Autodesk Inventor part; units mm, degrees
ref_plane "YZ Plane" through (0, 0, 0) normal (1, 0, 0) x (0, 1, 0)
ref_plane "XZ Plane" through (0, 0, 0) normal (0, 1, 0) x (-1, 0, 0)
ref_plane "XY Plane" through (0, 0, 0) normal (0, 0, 1) x (1, 0, 0)
sketch "Sketch1" plane through (0, 0, 0) normal (0, 1, 0) x (-1, 0, 0)
  line L0 (0, 0) -> (-2, 0)
  line L1 (-2, 0) -> (-3.1369, 0)
  line L2 (-3.1369, 0) -> (-3.1369, -16)
  line L3 (-3.1369, -16) -> (-1.7653, -16)
  line L4 (-1.7653, -16) -> (-1.7653, -18.3622)
  line L5 (-1.7653, -18.3622) -> (-3.1369, -18.3622)
  line L6 (-3.1369, -18.3622) -> (-3.1369, -19.3622)
  line L7 (-2, 0) -> (0, 0)
  line L8 (-2, 0) -> (0, 0)
  line L9 (-3.1369, -19.3622) -> (-3, -19.3622)
  line L10 (-3, -19.3622) -> (-3, -35.3622)
  line L11 (-3, -35.3622) -> (0, -35.3622)
  line L12 (0, -35.3622) -> (0, 0)
  dimension "d1" = 0
  dimension "d2" = 16
  dimension "d3" = 2.3622
  dimension "d6" = 3.1369
  dimension "d8" = 3
  dimension "d13" = 1
  dimension "d29" = 1.7653
  dimension "d30" = 16
revolve "Revolution1" add sketch "Sketch1" angle 360 about axis through (0, 0, -35.3622) along (0, 0, 1)
thread "Thread1"
sketch "Sketch3" plane through (0, 0, 0) normal (0, 0, 1) x (1, 0, 0)
  circle A0 centre (0, 0) radius 3.1369
  line L0 (-2.4166, -2) -> (2.4166, -2)
  line L1 (-2.5237, 1.8631) -> (2.5237, 1.8631)
  arc A1 (2.4166, -2) -> (2.5237, 1.8631) centre (0, 0) ccw
  arc A2 (-2.5237, 1.8631) -> (-2.4166, -2) centre (0, 0) ccw
  point P0 (0, 0)
  dimension "d36" = 5
extrude "Extrusion1" cut sketch "Sketch3" against normal blind 10 contours L1 A0
sketch "Sketch4" plane through (-2.5237, 1.8631, 0) normal (0, 1, 0) x (1, 0, 0)
  circle A0 centre (2.5237, 3) radius 1
  point P0 (2.5237, 0)
  dimension "d23" = 2
  dimension "d24" = 3
extrude "Extrusion2" cut sketch "Sketch4" against normal blind 10
thread "Thread2"
sketch "Sketch5" plane through (0, 0, -35.3622) normal (0, 0, -1) x (-1, 0, 0)
  circle A0 centre (0, 0) radius 3.1369
  line L0 (-2.5237, 1.8631) -> (2.5258, 1.8631)
  line L1 (2.5258, 1.8631) -> (2.5258, 4.5959)
  line L2 (2.5258, 4.5959) -> (-2.5237, 4.5959)
  line L3 (-2.5237, 4.5959) -> (-2.5237, 1.8631)
  point P0 (0, 0)
  dimension "d33" = 5
extrude "Extrusion3" cut sketch "Sketch5" against normal blind 16 contours L0 A0 | A0 L3 L2 L1 picked at (-0.6375, 2.3533)
properties part number "rod"
Geometry check sheet. Reference: the model listing, model coordinates, mm. A direction names the side the tool comes from. Give positions to 0.01 mm unless a question says otherwise; leave off trailing zeros. Order: outer loops, then holes, each group sorted by start corner. A loop starts at its lowest first (then second) coordinate and runs counter-clockwise, first axis right, second up. Notation, with made-up numbers: (-27, -11.5) - (2, -11.5) arc R7 cw to (2, -4.5) - close; hole circle Ø5 at (4, 49.5). An arc over 180 degrees is marked (long way). Write item = value, one per line. Start each with the question number.
1) Gauge pin test, flat ends, axial feed: pin 1 Ø3 at (x, y) = (-1, -0.5) entering from +Z; pin 2 Ø2.5 at (x, z) = (1, -28) entering from +Y; pin 3 Ø1 at (x, y) = (-1, 2.5) entering from +Z; pin 4 Ø1 at (x, z) = (-0.5, -24) entering from -Y. Record the tip position at first contact, or that the pin passes through.
2) Scan lines: L1, parallel to Z at x = -2.25, y = 0.5; L2, parallel to Z at x = -1.75, y = 2.5; L3, parallel to X at y = -0.6, z = -3. Record each from-to range of solid material in increasing order.
3) Section check B-B (y = 0). Enter the section's corners in (x, z).
4) Draft check along Z on faces 5 (the flat face through (0, -1, -35.362)), 6 (the flat face through (1.4, -1.4, -18.362)), 7 (the flat face through (0, -1, 0)), 8 (the flat face through (0, 1.863, -27)). Enter one of: released by +Z, released by -Z, zero draft, split by the parting line, or undercut.
5) Access from +Z, -Z, +X, -X, +Y, -Y to the whole of each face (thin tool, end or side, straight path). Record for faces 1 (the cylindrical face through (0, -3, -27)), 2 (the flat face through (0, 2.4, -10)), 3 (the cylindrical face through (-3.134, -0.138, -18.869)), 4 (the cylindrical face through (0.81, 1.57, -17.2)).
6) Section check C-C (y = 2.75). Enter the section's corners in (x, z).
7) Section check D-D (z = -15.5). Enter the section's corners in (x, y), then the cut area to 3 significant figures.
8) Section check A-A (x = 0). Enter the section's corners in (y, z).
Geometry check:
q1.pin_1 = 0
q1.pin_2 = 1.86
q1.pin_3 = -10
q1.pin_4 = -3
q2.L1 = -35.36 to -18.36, -16 to 0
q2.L2 = -19.36 to -18.36, -16 to -10
q2.L3 = -3.08 to -1, 1 to 3.08
q3.outline = (-3.14, -19.36) - (-3, -19.36) - (-3, -35.36) - (3, -35.36) - (3, -19.36) - (3.14, -19.36) - (3.14, -18.36) - (1.77, -18.36) - (1.77, -16) - (3.14, -16) - (3.14, 0) - (-3.14, 0) - (-3.14, -16) - (-1.77, -16) - (-1.77, -18.36) - (-3.14, -18.36) - close; hole circle Ø2 at (0, -3)
q4.face_5 = released by -Z
q4.face_6 = undercut
q4.face_7 = released by +Z
q4.face_8 = zero draft
q5.face_1 = -Z
q5.face_2 = +Z, +X, -X, +Y
q5.face_3 = +Z, -Z
q5.face_4 = none
q6.outline = (-1.51, -19.36) - (1.51, -19.36) - (1.51, -18.36) - (-1.51, -18.36) - close; (-1.51, -16) - (1.51, -16) - (1.51, -10) - (-1.51, -10) - close
q7.outline = circle Ø6.27 at (0, 0)
q7.area = 30.9 mm2
q8.outline = (-3.14, -19.36) - (-3, -19.36) - (-3, -35.36) - (1.86, -35.36) - (1.86, -19.36) - (3.14, -19.36) - (3.14, -18.36) - (1.77, -18.36) - (1.77, -16) - (3.14, -16) - (3.14, -10) - (1.86, -10) - (1.86, -4) - (-3.14, -4) - (-3.14, -16) - (-1.77, -16) - (-1.77, -18.36) - (-3.14, -18.36) - close; (-3.14, -2) - (1.86, -2) - (1.86, 0) - (-3.14, 0) - close
